Read the model definition and answer for the solid it produces. Units are mm, in the model's axes. A direction names the side the tool comes from. Coordinates: 2 decimals unless noted, no trailing zeros. Write each loop counter-clockwise with the first axis right and the second up, starting at its lowest first coordinate (ties: lowest second). Pieces come first, ordered by that corner, then holes.
1) The part is cut by section A-A (z = -8.5). Determine the outline of the cut face in (x, y).
2) The part is cut by section B-B (z = 8). Determine the outline of the cut face in (x, y), then the cut area to 3 significant figures.
3) Which of the six approach directions +Z, -Z, +X, -X, +Y, -Y give full straight-line access (tool end or side, diameter ignored) to faces 4 (the face through (6.763, 3.676, 17.535)), 5 (the face through (-7.51, 1.48, 8.37)), 6 (the face through (-9.4, 3, 9.4))?
4) Determine the mould class of faces 1 (the face through (7, 3, 15)), 2 (the face through (0, 2, -15)), 3 (the face through (20, 2, 2)) for opening direction X: +X half, -X half, draft (parallel to the pull), parting line (faces both ways), or undercut.
5) Find the intervals of material crossed by line 1 (X direction, y = 1.35, z = -13); line 2 (X direction, y = 4.6, z = -8.5); line 3 (Z direction, x = 8, y = 1.45), in increasing order.
6) Each of these flat-tipped pins is pushed along its axis until it touches: pin 1 Ø1.2 at (x, z) = (-9, -8.5) entering from +Y; pin 2 Ø1.6 at (x, z) = (8.5, 8.5) entering from -Y. Where does it stop, or does it pass through?
from build123d import *

# Parameters (mm, degrees)
SKETCH2_W           = 40
SKETCH2_H           = 30
SKETCH2_R           = 1
BOSS_EXTRUDE1_DEPTH = 5
SKETCH3_R           = 2
CUT_EXTRUDE1_DEPTH  = 2
SKETCH5_R           = 1
CUT_EXTRUDE2_DEPTH  = 26.495097568
SKETCH7_W           = 40
SKETCH7_H           = 5
BOSS_EXTRUDE2_DEPTH = 5
SKETCH8_R           = 1
CUT_EXTRUDE3_DEPTH  = 5


with BuildPart() as part:
    # Sketch2 → Boss-Extrude1 (new body)
    with BuildSketch(Plane(origin=(0, 0, 0), x_dir=(1, 0, 0), z_dir=(0, 1, 0))):
        Rectangle(SKETCH2_W, SKETCH2_H)
        with Locations(Location((-8.5, 8.5, 0), (0, 0, 270))):
            Circle(SKETCH2_R, mode=Mode.SUBTRACT)
        with Locations(Location((8.5, 8.5, 0), (0, 0, 270))):
            Circle(SKETCH2_R, mode=Mode.SUBTRACT)
        with Locations(Location((8.5, -8.5, 0), (0, 0, 270))):
            Circle(SKETCH2_R, mode=Mode.SUBTRACT)
        with Locations(Location((-8.5, -8.5, 0), (0, 0, 270))):
            Circle(SKETCH2_R, mode=Mode.SUBTRACT)
    extrude(amount=BOSS_EXTRUDE1_DEPTH)

    # Sketch3 → Cut-Extrude1 (cut)
    with BuildSketch(Plane(origin=(0, 5, 0), x_dir=(1, 0, 0), z_dir=(0, 1, 0))):
        with Locations(Location((-8.5, 8.5, 0), (0, 0, 270))):
            Circle(SKETCH3_R)
        with Locations(Location((8.5, 8.5, 0), (0, 0, 270))):
            Circle(SKETCH3_R)
        with Locations(Location((8.5, -8.5, 0), (0, 0, 270))):
            Circle(SKETCH3_R)
        with Locations(Location((-8.5, -8.5, 0), (0, 0, 270))):
            Circle(SKETCH3_R)
    extrude(amount=-CUT_EXTRUDE1_DEPTH, mode=Mode.SUBTRACT)

    # Sketch5 → Cut-Extrude2 (cut, through all)
    with BuildSketch(Plane.XZ):
        with Locations(Location((-7.5, -13, 0), (0, 0, 270))):
            Circle(SKETCH5_R)
        with Locations(Location((7.5, -13, 0), (0, 0, 270))):
            Circle(SKETCH5_R)
    extrude(amount=-CUT_EXTRUDE2_DEPTH, mode=Mode.SUBTRACT)

    # Sketch7 → Boss-Extrude2 (add)
    with BuildSketch(Plane.XY.offset(15)):
        with Locations((0, 2.5)):
            Rectangle(SKETCH7_W, SKETCH7_H)
    extrude(amount=BOSS_EXTRUDE2_DEPTH)

    # Sketch8 → Cut-Extrude3 (cut)
    with BuildSketch(Plane.XY.offset(20)):
        with Locations((-7.5, 3)):
            Circle(SKETCH8_R)
        with Locations((7.5, 3)):
            Circle(SKETCH8_R)
    extrude(amount=-CUT_EXTRUDE3_DEPTH, mode=Mode.SUBTRACT)


solid = part.part
Reported:
1. outline: (-20, 0) - (-9.5, 0) - (-9.5, 3) - (-10.5, 3) - (-10.5, 5) - (-20, 5) - close; (-7.5, 0) - (7.5, 0) - (7.5, 3) - (6.5, 3) - (6.5, 5) - (-6.5, 5) - (-6.5, 3) - (-7.5, 3) - close; (9.5, 0) - (20, 0) - (20, 5) - (10.5, 5) - (10.5, 3) - (9.5, 3) - close
2. outline: (-20, 0) - (-9.37, 0) - (-9.37, 3) - (-10.44, 3) - (-10.44, 5) - (-20, 5) - close; (-7.63, 0) - (7.63, 0) - (7.63, 3) - (6.56, 3) - (6.56, 5) - (-6.56, 5) - (-6.56, 3) - (-7.63, 3) - close; (9.37, 0) - (20, 0) - (20, 5) - (10.44, 5) - (10.44, 3) - (9.37, 3) - close
2. area: 174 mm2
3. face 4: +Z
3. face 5: +Y, -Y
3. face 6: +Y
4. face 1: undercut
4. face 2: draft
4. face 3: +X half
5. line 1: x = -20 to -8.5, -6.5 to 6.5, 8.5 to 20
5. line 2: x = -20 to -10.5, -6.5 to 6.5, 10.5 to 20
5. line 3: z = -15 to -13.87, -12.13 to -9.37, -7.63 to 7.63, 9.37 to 20
6. pin 1: stops at y = 3
6. pin 2: passes through
